Here's the drawing with two shaded views (mm, measured from the low corner). I have some questions. Round coordinates to 2 decimals unless told otherwise and drop trailing zeros. Loops run counter-clockwise (first coordinate to the right, second up) from the corner with the lowest first, then second, coordinate; pieces in that order, holes last. Notation, with made-up numbers: M 17,-40 L 55,-40 A18 cw 55,-21 Z; hole C -12,-3.75 d3. An arc over 180 degrees is marked long. One line per item, written item: value. Start each with the question number.
Q1. Imagine slicing it at B-B (y = 8.5). Please give me the cut outline in (x, z).
Q2. Please list where these lines run through material, in increasing order: line 1 along Y through (x, z) = (8.5, 26); line 2 along Z through (x, y) = (4.5, 13); line 3 along X through (y, z) = (8, 79.5).
Q3. Thinking about a two-plate mould opening in X: for the marked faces 1 and 2, which applies, released by +X, released by -X, zero draft, split by the parting line, or undercut?
Q4. I'm going to push flat-ended pins straight in: pin 1 Ø1 at (x, z) = (8.5, 41) entering from +Y; pin 2 Ø10 at (y, z) = (13.5, 45.5) entering from -X; pin 3 Ø3 at (y, z) = (3.5, 52) entering from +X. Where does each tip first touch, or does it pass through?
Q5. Imagine slicing it at A-A (x = 8.5). Please give me the cut outline in (y, z), then the cut area to 3 significant figures.
Q6. Imagine slicing it at C-C (z = 76). Please give me the cut outline in (x, y).
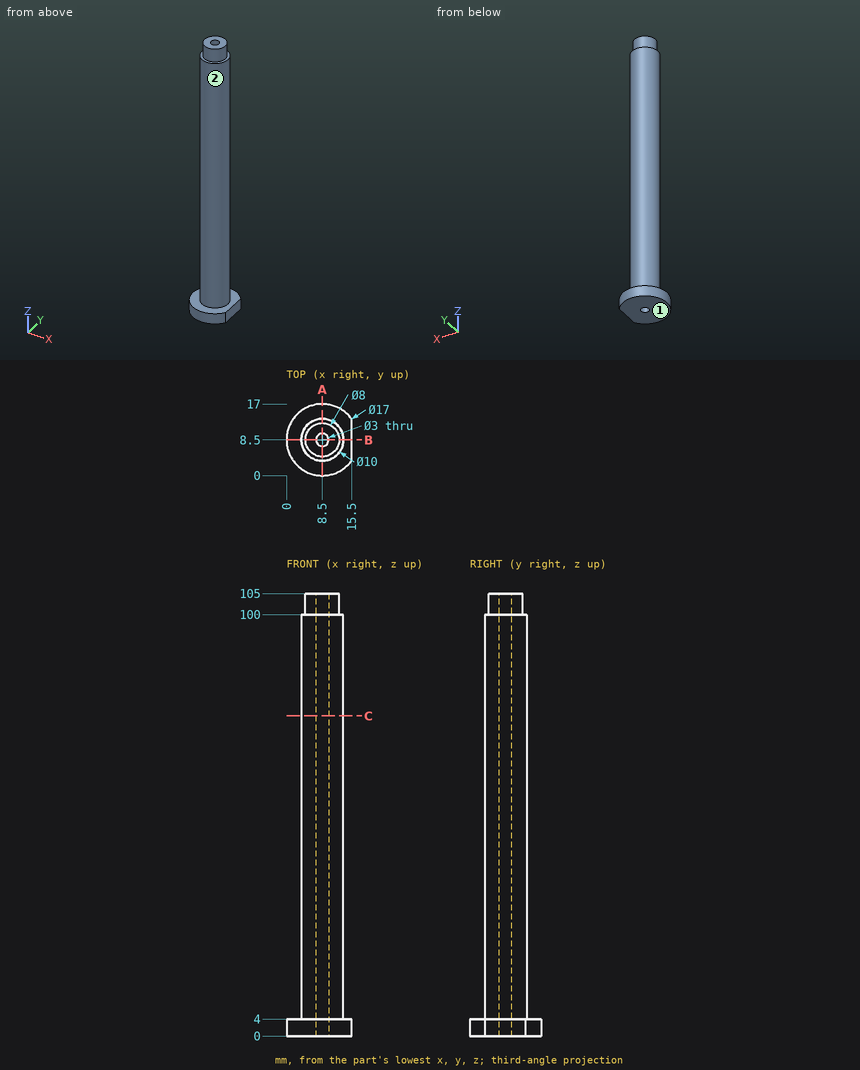
Report:
1. outline: M 0,0 L 7,0 L 7,105 L 4.5,105 L 4.5,100 L 3.5,100 L 3.5,4 L 0,4 Z; M 10,0 L 15.5,0 L 15.5,4 L 13.5,4 L 13.5,100 L 12.5,100 L 12.5,105 L 10,105 Z
2. line 1: y = 3.5 to 7, 10 to 13.5
2. line 2: z = 0 to 4
2. line 3: x = 3.53 to 7.09, 9.91 to 13.47
3. face 1: zero draft
3. face 2: split by the parting line
4. pin 1: stops at y = 13.5
4. pin 2: stops at x = 3.5
4. pin 3: stops at x = 12.07
5. outline: M 0,0 L 7,0 L 7,105 L 4.5,105 L 4.5,100 L 3.5,100 L 3.5,4 L 0,4 Z; M 10,0 L 17,0 L 17,4 L 13.5,4 L 13.5,100 L 12.5,100 L 12.5,105 L 10,105 Z
5. area: 753 mm²
6. outline: C 8.5,8.5 d10; hole C 8.5,8.5 d3
